Source: CAD feature listing. Evaluate the final solid. Frame: model axes, mm. A direction names the side the tool comes from. Give positions to 0.01 mm unless a question says otherwise; leave off trailing zeros. Loops run counter-clockwise (first coordinate to the right, second up) from the corner with the lowest first, then second, coordinate; pieces in that order, holes last. Notation, with made-up numbers: M -31,-39 L -21,-39 A30 cw -21,-10 Z; hole C 36,5.5 d5. An arc over 180 degrees is marked long. Put each result on its own line as item: value.
from build123d import *

# Parameters (mm, degrees)
SKETCH1_R               = 25.4
SKETCH1_R_2             = 22.225
BOSS_EXTRUDE1_DEPTH     = 914.4
CUT_EXTRUDE1_START      = -152.4
SKETCH2_R               = 25.4
CUT_EXTRUDE1_DEPTH      = 763.70528356
CUT_EXTRUDE2_DEPTH      = 148.321368528
SKETCH4_W               = 50.8
SKETCH4_H               = 16.486891384
CUT_EXTRUDE3_DEPTH      = 163.639355631
CUT_EXTRUDE4_REACH      = 151.106
CUT_EXTRUDE4_END_RADIUS = 22.225
SKETCH5_R               = 19.05


with BuildPart() as part:
    # Sketch1 → Boss-Extrude1 (new body)
    with BuildSketch(Plane.XY):
        Circle(SKETCH1_R)
        Circle(SKETCH1_R_2, mode=Mode.SUBTRACT)
    extrude(amount=BOSS_EXTRUDE1_DEPTH)

    # Sketch2 → Cut-Extrude1 (cut, through all)
    with BuildSketch(Plane(origin=(0, 0, 0), x_dir=(-1, 0, 0), z_dir=(0, 0, -1)).offset(CUT_EXTRUDE1_START)):
        Circle(SKETCH2_R)
    extrude(amount=-CUT_EXTRUDE1_DEPTH, mode=Mode.SUBTRACT)

    # Sketch3 → Cut-Extrude2 (cut, through all)
    with BuildSketch(Plane(origin=(0, 0, 9.525), x_dir=(-1, 0, 0), z_dir=(0, 0, -1))):
        with BuildLine():
            Line((-18.445083186, -17.4625), (18.445083186, -17.4625))
            ThreePointArc((18.445083186, -17.4625), (0, 25.4), (-18.445083186, -17.4625))
        make_face()
    extrude(amount=CUT_EXTRUDE2_DEPTH, mode=Mode.SUBTRACT)

    # Sketch4 → Cut-Extrude3 (cut, through all)
    with BuildSketch(Plane(origin=(0, 25.4, 0), x_dir=(1, 0, 0), z_dir=(0, 1, 0))):
        with Locations((0, -144.156554308)):
            Rectangle(SKETCH4_W, SKETCH4_H)
    extrude(amount=-CUT_EXTRUDE3_DEPTH, mode=Mode.SUBTRACT)

    # Cut-Extrude4: up to this cylinder (the profile starts outside it)
    cut_extrude4_end = Plane(origin=(0, 0, 108.847618), z_dir=(0, 0, -1)) * Cylinder(CUT_EXTRUDE4_END_RADIUS, 347.662, mode=Mode.PRIVATE)
    # Sketch5 → Cut-Extrude4 (cut, up to the surface)
    with BuildSketch(Plane(origin=(-17.960512242, -17.960512242, 0), x_dir=(0, 0, -1), z_dir=(-0.7071067811865464, -0.7071067811865488, 0)), mode=Mode.PRIVATE) as cut_extrude4_sk1:
        with Locations(Location((-108.847617901, 0, 0), (0, 0, 90))):
            Circle(SKETCH5_R)
    cut_extrude4_tool1 = extrude(cut_extrude4_sk1.sketch, amount=-CUT_EXTRUDE4_REACH, mode=Mode.PRIVATE) - cut_extrude4_end
    add(cut_extrude4_tool1.solids().sort_by_distance((-17.960512, -17.960512, 108.847618))[0], mode=Mode.SUBTRACT)


solid = part.part
1. Access query for faces 4 (the cylindrical face through (21.199, 6.676, 67.005)), 5 (the flat face through (-16, -17.462, 5)). Directions: +Z, -Z, +X, -X, +Y, -Y. A direction counts if a zero-diameter tool reaches every point of the face in a straight line with its end or side. Return the directions, or none.
Found:
face 4: +Z, -Z
face 5: -Z, +X, -X, +Y
2. Contact query for flat-ended pins moving along their axis: P1, Ø6, axis at y = 3.5, z = 20.5, coming from the -X side; P2, Ø8, axis at x = -13, z = 30.5, coming from the -Y side; P3, Ø1, axis at y = 10, z = 39, coming from the -X side. Output: stop coordinate, or through.
Found:
P1: x = -25.4
P2: y = -23.75
P3: x = -23.56
3. Material intervals for line 1 (Y direction, x = 0, z = 78) (3 decimals); line 2 (Y direction, x = 0, z = 103) (3 decimals), sorted ascending. Write a range as from..to.
Found:
line 1: -25.4..-22.225, 22.225..25.4
line 2: 22.225..25.4
4. Draft query along X for faces 1 (the cylindrical face through (-2.055, -24.778, 119.081)), 2 (the cylindrical face through (24.227, 7.629, 67.005)), 3 (the flat face through (0, -23, 0)). Return one class per face: pulls with the +X half, pulls with the -X half, needs draft (parallel to the pull), parting line crosses it, or undercut.
Found:
face 1: undercut
face 2: parting line crosses it
face 3: needs draft
5. Section query D-D (y = 16). Output: boundary loops of the cut face in (x, z) (3 decimals), plus the area to 3 significant figures.
Found:
outline: M -19.727,9.525 L -15.426,9.525 L -15.426,135.913 L -19.727,135.913 Z; M 15.426,9.525 L 19.727,9.525 L 19.727,135.913 L 15.426,135.913 Z
area: 1,090 mm^2
6. Section query B-B (z = 73). Output: boundary loops of the cut face in (x, y) (3 decimals).
Found:
outline: C 0,0 d50.8; hole C 0,0 d44.45
7. Section query A-A (y = 9). Output: boundary loops of the cut face in (x, z) (3 decimals).
Found:
outline: M -23.752,9.525 L -20.321,9.525 L -20.321,135.913 L -23.752,135.913 Z; M 20.321,9.525 L 23.752,9.525 L 23.752,135.913 L 20.321,135.913 Z
8. Section query C-C (x = -2.5). State how many separate pieces and enclosed holes the cut face has, plus the area to 3 significant figures.
Found:
separate pieces: 3
enclosed holes: 0
area: 763 mm^2
